from build123d import *

# Parameters (mm, degrees)
ESQUISSE1_R             = 2.5
BOSS_EXTRU_1_DEPTH      = 4
ESQUISSE2_R             = 2.1
ESQUISSE2_R_2           = 2
ENL_V_MAT_EXTRU_1_DEPTH = 4
BOSS_EXTRU_2_DEPTH      = 6
CONG_1_R                = 2


with BuildPart() as part:
    # Esquisse1 → Boss.-Extru.1 (new body)
    with BuildSketch(Plane(origin=(0, 0, 0), x_dir=(1, 0, 0), z_dir=(0, 1, 0))):
        Polygon((0, 218), (0, 186), (9, 186), (9, 32), (0, 32), (0, 0), (32, 0), (32, 9), (186, 9), (186, 0), (218, 0), (218, 32), (209, 32), (209, 186), (218, 186), (218, 218), (186, 218), (186, 209), (32, 209), (32, 218), align=None)
        with Locations(Location((8, 210, 0), (0, 0, 270))):
            Circle(ESQUISSE1_R, mode=Mode.SUBTRACT)
        with Locations(Location((210, 210, 0), (0, 0, 270))):
            Circle(ESQUISSE1_R, mode=Mode.SUBTRACT)
        with Locations(Location((210, 8, 0), (0, 0, 270))):
            Circle(ESQUISSE1_R, mode=Mode.SUBTRACT)
        with Locations(Location((8, 8, 0), (0, 0, 270))):
            Circle(ESQUISSE1_R, mode=Mode.SUBTRACT)
    extrude(amount=BOSS_EXTRU_1_DEPTH)

    # Esquisse2 → Enlèv. mat.-Extru.1 (cut)
    with BuildSketch(Plane(origin=(0, 4, 0), x_dir=(1, 0, 0), z_dir=(0, 1, 0))):
        with Locations(Location((172.5, 22.6, 0), (0, 0, 90))):
            Circle(ESQUISSE2_R)
        with Locations(Location((153, 82, 0), (0, 0, 90))):
            Circle(ESQUISSE2_R)
        with Locations(Location((20, 107, 0), (0, 0, 90))):
            Circle(ESQUISSE2_R)
        with Locations(Location((49, 122.5, 0), (0, 0, 270))):
            Circle(ESQUISSE2_R_2)
        with Locations(Location((144, 122.5, 0), (0, 0, 270))):
            Circle(ESQUISSE2_R_2)
        with Locations(Location((144, 145, 0), (0, 0, 270))):
            Circle(ESQUISSE2_R_2)
        with Locations(Location((49, 145, 0), (0, 0, 270))):
            Circle(ESQUISSE2_R_2)
        with Locations(Location((67.6, 199.5, 0), (0, 0, 270))):
            Circle(ESQUISSE2_R_2)
        with Locations(Location((67.6, 150.9, 0), (0, 0, 270))):
            Circle(ESQUISSE2_R_2)
        with Locations(Location((125.4, 150.9, 0), (0, 0, 90))):
            Circle(ESQUISSE2_R_2)
        with Locations(Location((125.4, 199.5, 0), (0, 0, 90))):
            Circle(ESQUISSE2_R_2)
    extrude(amount=-ENL_V_MAT_EXTRU_1_DEPTH, mode=Mode.SUBTRACT)

    # Esquisse4 → Boss.-Extru.2 (add)
    with BuildSketch(Plane(origin=(0, 4, 0), x_dir=(1, 0, 0), z_dir=(0, 1, 0))):
        Polygon((198.7, 14.3), (183.7, 14.3), (183.7, 19.3), (196.353215425, 19.3), (198.7, 21.646784575), (198.7, 34.3), (203.7, 34.3), (203.7, 19.3), align=None)
        Polygon((19.3, 203.7), (34.3, 203.7), (34.3, 198.7), (21.646784575, 198.7), (19.3, 196.353215425), (19.3, 183.7), (14.3, 183.7), (14.3, 198.7), align=None)
        Polygon((203.7, 198.7), (203.7, 183.7), (198.7, 183.7), (198.7, 196.353215425), (196.353215425, 198.7), (183.7, 198.7), (183.7, 203.7), (198.7, 203.7), align=None)
    extrude(amount=BOSS_EXTRU_2_DEPTH)

    # Congé1
    cong_1_edges = [part.edges().sort_by_distance(p)[0] for p in [
        (0, 2, 0),
        (0, 2, -32),
        (9, 2, -32),
        (9, 2, -186),
        (0, 2, -186),
        (0, 2, -218),
        (32, 2, -218),
        (32, 2, -209),
        (186, 2, -209),
        (186, 2, -218),
        (218, 2, -218),
        (218, 2, -186),
        (209, 2, -186),
        (209, 2, -32),
        (218, 2, -32),
        (218, 2, 0),
        (186, 2, 0),
        (186, 2, -9),
        (32, 2, -9),
        (32, 2, 0),
    ]]
    fillet(cong_1_edges, radius=CONG_1_R)


solid = part.part
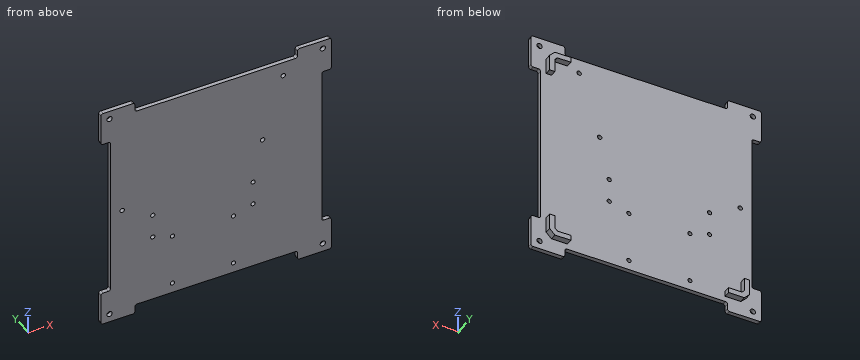
Design review of the part built by this model. Coordinates are the model's own, in mm. Round coordinates to 2 decimals unless told otherwise and drop trailing zeros. Write each loop counter-clockwise with the first axis right and the second up, starting at its lowest first coordinate (ties: lowest second). Pieces come first, ordered by that corner, then holes.
Item 1: Consider section B-B on x = 78. Give the boundary of the cut face in (y, z), and give its area (3 significant figures).
Item 2: Wall thickness on L1, parallel to X at y = 2.6, z = -150.9; L2, parallel to Z at x = 125.4, y = 2.6; L3, parallel to Z at x = 144, y = 1.2: over which ranges is each line inside the solid? List them lowest first.
Item 3: For pin 1 Ø3 at (x, y) = (92, 3.5) entering from +Z; pin 2 Ø4.5 at (x, z) = (8, -8) entering from +Y; pin 3 Ø3 at (y, z) = (2.5, -112) entering from +X; pin 4 Ø1 at (y, z) = (3.5, -163) entering from -X, all flat-tipped, find the tip position at first contact; note any pin that passes through.
Item 4: Consider section C-C on z = -172. Give the boundary of the cut face in (x, y).
Item 5: Consider section A-A on y = 7. Give the boundary of the cut face in (x, z).
Check values:
1. outline: (0, -209) - (4, -209) - (4, -9) - (0, -9) - close
1. area: 800 mm2
2. L1: x = 9 to 65.6, 69.6 to 123.4, 127.4 to 209
2. L2: z = -209 to -201.5, -197.5 to -152.9, -148.9 to -9
2. L3: z = -209 to -147, -143 to -124.5, -120.5 to -9
3. pin 1: stops at z = -9
3. pin 2: passes through
3. pin 3: stops at x = 209
3. pin 4: stops at x = 9
4. outline: (9, 0) - (209, 0) - (209, 4) - (9, 4) - close
5. outline: (14.3, -198.7) - (19.3, -203.7) - (34.3, -203.7) - (34.3, -198.7) - (21.65, -198.7) - (19.3, -196.35) - (19.3, -183.7) - (14.3, -183.7) - close; (183.7, -203.7) - (198.7, -203.7) - (203.7, -198.7) - (203.7, -183.7) - (198.7, -183.7) - (198.7, -196.35) - (196.35, -198.7) - (183.7, -198.7) - close; (183.7, -19.3) - (196.35, -19.3) - (198.7, -21.65) - (198.7, -34.3) - (203.7, -34.3) - (203.7, -19.3) - (198.7, -14.3) - (183.7, -14.3) - close
